from build123d import *

# Parameters (mm, degrees)
SKETCH1_R           = 1.75
BOSS_EXTRUDE1_DEPTH = 3


with BuildPart() as part:
    # Sketch1 → Boss-Extrude1 (new body)
    with BuildSketch(Plane(origin=(0, 0, 0), x_dir=(1, 0, 0), z_dir=(0, 1, 0))):
        Polygon((-73.5, 33), (-44.1, 33), (-44.1, 36), (-14.7, 36), (-14.7, 33), (-5, 33), (-5, 32), (-5, 29), (0, 29), (5, 29), (5, 33), (14.7, 33), (14.7, 36), (44.1, 36), (44.1, 33), (73.5, 33), (73.5, 36), (76.5, 36), (76.5, 20.4), (73.5, 20.4), (73.5, 4.8), (76.5, 4.8), (76.5, -10.8), (73.5, -10.8), (73.5, -26.4), (76.5, -26.4), (76.5, -42), (-76.5, -42), (-76.5, -26.4), (-73.5, -26.4), (-73.5, -10.8), (-76.5, -10.8), (-76.5, 4.8), (-73.5, 4.8), (-73.5, 20.4), (-76.5, 20.4), (-76.5, 36), (-73.5, 36), align=None)
        with Locations((-56.2, -8)):
            Circle(SKETCH1_R, mode=Mode.SUBTRACT)
        with Locations((-55.2, 20)):
            Circle(SKETCH1_R, mode=Mode.SUBTRACT)
        with Locations((49.8, 20)):
            Circle(SKETCH1_R, mode=Mode.SUBTRACT)
        with Locations((55.5, -8)):
            Circle(SKETCH1_R, mode=Mode.SUBTRACT)
    extrude(amount=BOSS_EXTRUDE1_DEPTH)


solid = part.part
Geometry check sheet. Reference: the model listing, model coordinates, mm. A direction names the side the tool comes from. Round coordinates to 2 decimals unless told otherwise and drop trailing zeros. Write each loop counter-clockwise with the first axis right and the second up, starting at its lowest first coordinate (ties: lowest second). Pieces come first, ordered by that corner, then holes.
Item 1: Mould release check, pull along Z, two halves, no side actions. Record for faces 4 (the face through (-73.5, 1, -35)), 5 (the face through (1, 1, 42)), 6 (the face through (75, 1, 10.8)), 7 (the face through (-75, 1, 26.4)): +Z half, -Z half, draft (parallel to the pull), parting line (faces both ways), or undercut.
Determined:
face 4: draft
face 5: +Z half
face 6: undercut
face 7: undercut
Item 2: Go/stop test with flat-tipped pins: pin 1 Ø1.5 at (y, z) = (1, -14.5) entering from +X; pin 2 Ø0.9 at (x, y) = (-11.5, 2) entering from -Z; pin 3 Ø0.9 at (y, z) = (1, -15) entering from -X. Record where each tip stops, or that it passes through.
Determined:
pin 1: stops at x = 73.5
pin 2: stops at z = -33
pin 3: stops at x = -73.5
Item 3: Section check A-A (x = 49.8). Record the boundary of the cut face in (y, z).
Determined:
outline: (0, -33) - (3, -33) - (3, -21.75) - (0, -21.75) - close; (0, -18.25) - (3, -18.25) - (3, 42) - (0, 42) - close
Item 4: Access from +Z, -Z, +X, -X, +Y, -Y to the whole of each face (thin tool, end or side, straight path). Record for faces 1 (the face through (5, 1, -31)), 2 (the face through (-75, 1, -4.8)), 3 (the face through (75, 1, -20.4)).
Determined:
face 1: -Z, +Y, -Y
face 2: -X, +Y, -Y
face 3: +X, +Y, -Y
Item 5: Section check C-C (y = 1.9). Give the number of separate pieces and of enclosed holes in the cut face, plus the area to 3 significant figures.
Determined:
separate pieces: 1
enclosed holes: 4
area: 11,400 mm2
Item 6: Section check D-D (x = -12). Record the boundary of the cut face in (y, z), plus the area to 3 significant figures.
Determined:
outline: (0, -33) - (3, -33) - (3, 42) - (0, 42) - close
area: 225 mm2
Item 7: Material ranges on line 1 along X through (y, z) = (0.6, 8); line 2 along Z through (x, y) = (49.8, 1.7); line 3 along X through (y, z) = (1, -20), recorded low to high.
Determined:
line 1: x = -76.5 to -57.95, -54.45 to 53.75, 57.25 to 76.5
line 2: z = -33 to -21.75, -18.25 to 42
line 3: x = -73.5 to -56.95, -53.45 to 48.05, 51.55 to 73.5
Item 8: Section check B-B (z = 8). Record the boundary of the cut face in (x, y), plus the area to 3 significant figures.
Determined:
outline: (-76.5, 0) - (-57.95, 0) - (-57.95, 3) - (-76.5, 3) - close; (-54.45, 0) - (53.75, 0) - (53.75, 3) - (-54.45, 3) - close; (57.25, 0) - (76.5, 0) - (76.5, 3) - (57.25, 3) - close
area: 438 mm2
